The listing builds one solid part. Answer for the finished solid, in the listing's coordinates (mm). A direction names the side the tool comes from. Round coordinates to 2 decimals unless told otherwise and drop trailing zeros. Order: outer loops, then holes, each group sorted by start corner. A loop starts at its lowest first (then second) coordinate and runs counter-clockwise, first axis right, second up. Notation, with made-up numbers: (85, 85.25) -> (136, 85.25) arc R19 ccw to (136, 107.25) -> close; hole circle Ø8 at (-1.5, 6). An arc over 180 degrees is marked (long way). Return JSON: item names as keys, results as strings. Group by question number.
(1) Each of these flat-tipped pins is pushed along its axis until it touches: pin 1 (2 mm diameter, centred on x = -145.79, y = 238.73, fed in from -Z); pin 2 (1.5 mm diameter, centred on y = 159.5, z = 16.5, fed in from -X); pin 3 (6 mm diameter, centred on y = 182, z = 6, fed in from -X); pin 4 (4 mm diameter, centred on y = 193, z = 6, fed in from -X). Where does it stop, or does it pass through?
(2) Determine the mould class of faces 4 (the face through (-197.377, 157.691, 2.69)), 5 (the face through (-179.44, 163.64, 2.93)), 6 (the face through (-174.265, 156.048, 9.658)) for opening direction Z: +Z half, -Z half, draft (parallel to the pull), parting line (faces both ways), or undercut.
(3) The part is cut by section A-A (y = 196). Determine the outline of the cut face in (x, z) (3 decimals), plus the area to 3 significant figures.
(4) Consider line 1 (Z direction, x = -189.5, y = 175) (3 decimals); line 2 (Y direction, x = -176, z = 6.5); line 3 (X direction, y = 154, z = 16.25). Determine where each line is inside the solid, lowest interval first. Write a range as [from, to].
(5) The part is cut by section B-B (x = -146). Determine the outline of the cut face in (y, z), plus the area to 3 significant figures.
(6) Which of the six approach directions +Z, -Z, +X, -X, +Y, -Y give full straight-line access (tool end or side, diameter ignored) to faces 1 (the face through (-186, 161, 2.025)), 2 (the face through (-197.531, 157.691, 16.213)), 3 (the face through (-125.585, 155, 9))?
(7) The part is cut by section C-C (z = 8). Count the separate pieces of the cut face and the enclosed holes in it, plus the area to 3 significant figures.
from build123d import *

# Parameters (mm, degrees)
BOSS_EXTRUDE1_DEPTH = 19.05
SKETCH2_R           = 1.7
CUT_EXTRUDE1_DEPTH  = 302.810637772
CUT_EXTRUDE2_DEPTH  = 302.810637772
BOSS_EXTRUDE2_DEPTH = 135
BOSS_EXTRUDE3_START = -19.05
BOSS_EXTRUDE3_DEPTH = 19.05
CUT_EXTRUDE4_DEPTH  = 316.043777756
CUT_EXTRUDE5_DEPTH  = 249.524391307
FILLET2_R           = 50
FILLET3_R           = 10
FILLET4_R           = 3
SKETCH8_R           = 3
CUT_EXTRUDE6_DEPTH  = 316.015975709


with BuildPart() as part:
    # Sketch1 → Boss-Extrude1 (new body)
    with BuildSketch(Plane.XY):
        with BuildLine():
            Line((-179.085368151, -18.789194183), (-179.085368151, 212.188334746))
            ThreePointArc((-179.085368151, 212.188334746), (-149.085368151, 242.188334746), (-119.085368151, 212.188334746))
            Line((-119.085368151, 212.188334746), (-119.085368151, -18.789194183))
            ThreePointArc((-119.085368151, -18.789194183), (-149.085368151, -48.789194183), (-179.085368151, -18.789194183))
        make_face()
        with BuildLine():
            Line((-172.585368151, -18.789194183), (-172.585368151, 212.188334746))
            ThreePointArc((-172.585368151, 212.188334746), (-149.085368151, 235.688334746), (-125.585368151, 212.188334746))
            Line((-125.585368151, 212.188334746), (-125.585368151, -18.789194183))
            ThreePointArc((-125.585368151, -18.789194183), (-149.085368151, -42.289194183), (-172.585368151, -18.789194183))
        make_face(mode=Mode.SUBTRACT)
    extrude(amount=BOSS_EXTRUDE1_DEPTH)

    # Sketch2 → Cut-Extrude1 (cut, through all)
    with BuildSketch(Plane.XY.offset(19.05)):
        with Locations((-145.785368151, 238.734002942)):
            Circle(SKETCH2_R)
        with Locations((-122.335368151, 212.188334746)):
            Circle(SKETCH2_R)
        with Locations((-152.485368151, -45.322239617)):
            Circle(SKETCH2_R)
        with Locations((-168.000474547, -37.70430058)):
            Circle(SKETCH2_R)
        with Locations((-175.835368151, -18.789194183)):
            Circle(SKETCH2_R)
        with Locations((-175.835368151, 212.188334746)):
            Circle(SKETCH2_R)
        with Locations((-145.685368151, -45.322239617)):
            Circle(SKETCH2_R)
        with Locations((-175.835368151, 100.099570281)):
            Circle(SKETCH2_R)
        with Locations((-175.835368151, 93.299570281)):
            Circle(SKETCH2_R)
        with Locations((-122.335368151, 100.099570281)):
            Circle(SKETCH2_R)
        with Locations((-122.335368151, 93.299570281)):
            Circle(SKETCH2_R)
        with Locations((-122.335368151, -18.789194183)):
            Circle(SKETCH2_R)
        with Locations((-130.170261754, -37.70430058)):
            Circle(SKETCH2_R)
        with Locations((-175.835368151, 156.699570281)):
            Circle(SKETCH2_R)
        with Locations((-122.335368151, 156.699570281)):
            Circle(SKETCH2_R)
        with Locations((-175.835368151, 66.699570281)):
            Circle(SKETCH2_R)
        with Locations((-122.335368151, 66.699570281)):
            Circle(SKETCH2_R)
        with Locations((-175.835368151, 36.699570281)):
            Circle(SKETCH2_R)
        with Locations((-122.335368151, 36.699570281)):
            Circle(SKETCH2_R)
        with Locations((-175.835368151, 6.699570281)):
            Circle(SKETCH2_R)
        with Locations((-122.335368151, 6.699570281)):
            Circle(SKETCH2_R)
        with Locations((-152.385368151, 238.734002942)):
            Circle(SKETCH2_R)
    extrude(amount=-CUT_EXTRUDE1_DEPTH, mode=Mode.SUBTRACT)

    # Sketch3 → Cut-Extrude2 (cut, through all)
    with BuildSketch(Plane.XY.offset(19.05)):
        Polygon((-149.085368151, 96.699570281), (-100.167336626, 96.699570281), (-100.167336626, -59.171887956), (-212.527814826, -59.171887956), (-212.527814826, 96.699570281), align=None)
    extrude(amount=-CUT_EXTRUDE2_DEPTH, mode=Mode.SUBTRACT)

    # Sketch4 → Boss-Extrude2 (add)
    with BuildSketch(Plane.XZ.offset(-96.699570281)):
        with BuildLine():
            Line((-179.085368151, 19.05), (-196.652205402, 19.05))
            ThreePointArc((-196.652205402, 19.05), (-200.585368151, 9.525), (-196.652205402, 0))
            Line((-196.652205402, 0), (-179.085368151, 0))
            Line((-179.085368151, 0), (-179.085368151, 19.05))
        make_face()
    extrude(amount=-BOSS_EXTRUDE2_DEPTH)

    # Sketch5 → Boss-Extrude3 (add)
    with BuildSketch(Plane.XY.offset(19.05).offset(BOSS_EXTRUDE3_START)):
        with BuildLine():
            Line((-179.085368151, 231.699570281), (-179.085368151, 212.188334746))
            ThreePointArc((-179.085368151, 212.188334746), (-174.234371945, 228.544605963), (-161.250194275, 239.611263206))
            Line((-161.250194275, 239.611263206), (-179.085368151, 231.699570281))
        make_face()
    extrude(amount=BOSS_EXTRUDE3_DEPTH)

    # Sketch6 → Cut-Extrude4 (cut, through all)
    with BuildSketch(Plane.XY.offset(19.05)):
        with BuildLine():
            Line((-170.167781213, 235.655416744), (-200.585368151, 235.655416744))
            Line((-200.585368151, 235.655416744), (-200.585368151, 214.140637656))
            add(Edge.make_bspline(
                [(-170.167781213, 235.655416744), (-176.900282948, 230.746544465), (-186.999558372, 219.576390382), (-197.475317375, 218.661877457), (-200.585368151, 214.140637656)],
                knots=[0, 0, 0, 0, 0.548460348, 1, 1, 1, 1], degree=3))
        make_face()
    extrude(amount=-CUT_EXTRUDE4_DEPTH, mode=Mode.SUBTRACT)

    # Sketch7 → Cut-Extrude5 (cut, through all)
    with BuildSketch(Plane.XZ.offset(-96.699570281)):
        with BuildLine():
            Line((-190.585368151, 17.025), (-178.585368151, 17.025))
            Line((-178.585368151, 17.025), (-178.585368151, 2.025))
            Line((-178.585368151, 2.025), (-190.585368151, 2.025))
            ThreePointArc((-190.585368151, 2.025), (-198.085368151, 9.525), (-190.585368151, 17.025))
        make_face()
    extrude(amount=-CUT_EXTRUDE5_DEPTH, mode=Mode.SUBTRACT)

    # Fillet2
    fillet2_edges = [part.edges().sort_by_distance(p)[0] for p in [
        (-170.167781213, 235.655416744, 9.525),
    ]]
    fillet(fillet2_edges, radius=FILLET2_R)

    # Fillet3
    # the kernel refuses this fillet: 10 mm, written as the material it takes off along each edge
    with BuildSketch(Plane(origin=(-196.652205402, 66.752998532, 0), x_dir=(1, 0, 0), z_dir=(0, 1, 0))) as fillet3_piece_1:
        with BuildLine():
            CenterArc((6.099219193, -10), FILLET3_R, 90, 97.799925588)
            ThreePointArc((-3.808260974, -11.357142857), (-3.23274377, -5.233062714), (0, 0))
            Line((0, 0), (6.099219193, 0))
        make_face()
    extrude(amount=180.922793438, mode=Mode.SUBTRACT)
    with BuildSketch(Plane(origin=(-196.652205402, 66.752998532, 19.05), x_dir=(-0.3179212804444137, 0, -0.9481171127242586), z_dir=(0, 1, 0))) as fillet3_piece_2:
        with BuildLine():
            CenterArc((7.542099552, -8.961986896), FILLET3_R, 63.66281519, 97.799925588)
            Line((-1.939071576, -5.782774091), (0, 0))
            ThreePointArc((0, 0), (5.98931435, 1.401317691), (11.9786287, 0))
        make_face()
    extrude(amount=180.922793438, mode=Mode.SUBTRACT)

    # Fillet4
    fillet4_edges = [part.edges().sort_by_distance(p)[0] for p in [
        (-178.585368151, 162.718537025, 17.025),
        (-178.585368151, 162.718537025, 2.025),
    ]]
    fillet(fillet4_edges, radius=FILLET4_R)

    # Sketch8 → Cut-Extrude6 (cut, through all)
    with BuildSketch(Plane(origin=(0, 0, 0), x_dir=(-1, 0, 0), z_dir=(0, 0, -1))):
        with Locations((187.552986209, 211.995977711)):
            Circle(SKETCH8_R)
    extrude(amount=-CUT_EXTRUDE6_DEPTH, mode=Mode.SUBTRACT)


solid = part.part
Answer below:
{
 "1": {"pin 1": "passes through", "pin 2": "stops at x = -197.98", "pin 3": "stops at x = -200.5", "pin 4": "stops at x = -200.35"},
 "2": {"face 4": "-Z half", "face 5": "undercut", "face 6": "draft"},
 "3": {"outline": "(-200.542, 9.525) arc R10 ccw to (-190.553, 0) -> (-172.585, 0) -> (-172.585, 19.05) -> (-190.553, 19.05) arc R10 ccw to start; (-125.585, 0) -> (-119.085, 0) -> (-119.085, 19.05) -> (-125.585, 19.05) -> close; hole (-190.585, 2.025) -> (-181.585, 2.025) arc R3 ccw to (-178.585, 5.025) -> (-178.585, 14.025) arc R3 ccw to (-181.585, 17.025) -> (-190.585, 17.025) arc R7.5 ccw to start", "area": "349 mm²"},
 "4": {"line 1": "z = [0, 2.025], [17.025, 19.05]", "line 2": "y = [96.7, 98.41], [101.79, 155.01], [158.39, 210.5], [213.88, 230.97]", "line 3": "x = [-197.49, -193.91], [-179.57, -172.59], [-125.59, -119.09]"},
 "5": {"outline": "(235.48, 0) -> (237.05, 0) -> (237.05, 19.05) -> (235.48, 19.05) -> close; (240.42, 0) -> (242.03, 0) -> (242.03, 19.05) -> (240.42, 19.05) -> close", "area": "60.4 mm²"},
 "6": {"face 1": "+Y, -Y", "face 2": "+Z, -X, +Y, -Y", "face 3": "+Z, -Z, -Y"},
 "7": {"separate pieces": "2", "enclosed holes": "8", "area": "2,250 mm²"}
}
